```python
from build123d import *

# Parameters (mm, degrees)
SKETCH9_R            = 30
BOSS_EXTRUDE11_DEPTH = 180
SKETCH10_W           = 35
SKETCH10_H           = 25
BOSS_EXTRUDE12_DEPTH = 20
SKETCH11_R           = 7.5
CUT_EXTRUDE2_DEPTH   = 201
SHELL1_T             = -1


with BuildPart() as part:
    # Sketch9 → Boss-Extrude11 (new body)
    with BuildSketch(Plane.XY):
        Circle(SKETCH9_R)
    extrude(amount=BOSS_EXTRUDE11_DEPTH)

    # Sketch10 → Boss-Extrude12 (add)
    with BuildSketch(Plane.XY.offset(180)):
        Rectangle(SKETCH10_W, SKETCH10_H)
    extrude(amount=BOSS_EXTRUDE12_DEPTH)

    # Sketch11 → Cut-Extrude2 (cut, through all)
    with BuildSketch(Plane.XY.offset(200)):
        Circle(SKETCH11_R)
    extrude(amount=-CUT_EXTRUDE2_DEPTH, mode=Mode.SUBTRACT)

    # Shell1
    shell1_openings = [part.faces().sort_by_distance(p)[0] for p in [
        (7.5, 0, 0),
    ]]
    offset(amount=SHELL1_T, openings=shell1_openings, kind=Kind.INTERSECTION)


solid = part.part
```
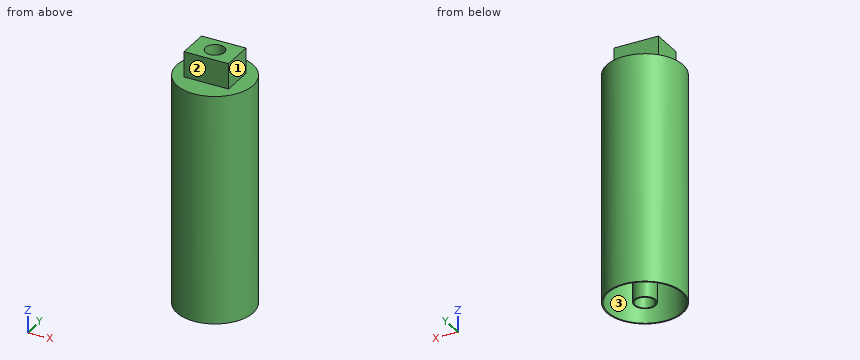
Verification items for the finished model (mm, model axes). Face numbers are marked on the shaded views. Give positions to 0.01 mm unless a question says otherwise; leave off trailing zeros. Loops run counter-clockwise (first coordinate to the right, second up) from the corner with the lowest first, then second, coordinate; pieces in that order, holes last.
1. Section check C-C, the plane z = 91. Enter the section's corners in (x, y), then the cut area to 3 significant figures.
2. Section check D-D, the plane x = -23. Enter the section's corners in (y, z), then the cut area to 3 significant figures.
3. Go/stop test with flat-tipped pins: pin 1 Ø10 at (x, z) = (5.5, 188) entering from -Y; pin 2 Ø9 at (x, y) = (0, 0) entering from -Z; pin 3 Ø10 at (y, z) = (19.5, 57) entering from +X; pin 4 Ø17.5 at (x, y) = (-2.5, 4.5) entering from -Z. Record where each tip stops, or that it passes through.
4. Section check B-B, the plane y = 0. Enter the section's corners in (x, z).
5. Section check A-A, the plane x = 0. Enter the section's corners in (y, z), then the cut area to 3 significant figures.
6. Thickness scan on line 1 (Y direction, x = 0, z = 150); line 2 (Y direction, x = -2.5, z = 82); line 3 (X direction, y = -1.5, z = 94.5). Record the ranges inside material, lowest first.
7. Mould release check, pull along Y, two halves, no side actions. Record for the marked faces 1, 2 and 3: released by +Y, released by -Y, zero draft, split by the parting line, or undercut.
Geometry says:
1. outline: circle Ø60 at (0, 0); circle Ø17 at (0, 0); hole circle Ø58 at (0, 0); hole circle Ø15 at (0, 0)
1. area: 236 mm2
2. outline: (-19.26, 0) - (-17.66, 0) - (-17.66, 179) - (17.66, 179) - (17.66, 0) - (19.26, 0) - (19.26, 180) - (-19.26, 180) - close
2. area: 611 mm2
3. pin 1: stops at y = -12.5
3. pin 2: passes through
3. pin 3: stops at x = 26.26
3. pin 4: stops at z = 0
4. outline: (-30, 0) - (-29, 0) - (-29, 179) - (-16.5, 179) - (-16.5, 199) - (-8.5, 199) - (-8.5, 0) - (-7.5, 0) - (-7.5, 200) - (-17.5, 200) - (-17.5, 180) - (-30, 180) - close; (7.5, 0) - (8.5, 0) - (8.5, 199) - (16.5, 199) - (16.5, 179) - (29, 179) - (29, 0) - (30, 0) - (30, 180) - (17.5, 180) - (17.5, 200) - (7.5, 200) - close
5. outline: (-30, 0) - (-29, 0) - (-29, 179) - (-11.5, 179) - (-11.5, 199) - (-8.5, 199) - (-8.5, 0) - (-7.5, 0) - (-7.5, 200) - (-12.5, 200) - (-12.5, 180) - (-30, 180) - close; (7.5, 0) - (8.5, 0) - (8.5, 199) - (11.5, 199) - (11.5, 179) - (29, 179) - (29, 0) - (30, 0) - (30, 180) - (12.5, 180) - (12.5, 200) - (7.5, 200) - close
5. area: 841 mm2
6. line 1: y = -30 to -29, -8.5 to -7.5, 7.5 to 8.5, 29 to 30
6. line 2: y = -29.9 to -28.89, -8.12 to -7.07, 7.07 to 8.12, 28.89 to 29.9
6. line 3: x = -29.96 to -28.96, -8.37 to -7.35, 7.35 to 8.37, 28.96 to 29.96
7. face 1: zero draft
7. face 2: released by -Y
7. face 3: undercut
